Autodesk Inventor part; units mm, degrees
ref_plane "YZ Plane" through (0, 0, 0) normal (1, 0, 0) x (0, 1, 0)
ref_plane "XZ Plane" through (0, 0, 0) normal (0, 1, 0) x (-1, 0, 0)
ref_plane "XY Plane" through (0, 0, 0) normal (0, 0, 1) x (1, 0, 0)
sketch "Sketch1" plane through (0, 0, 0) normal (0, 1, 0) x (-1, 0, 0)
  line L0 (0, 0) -> (83.3, 0)
  line L1 (83.3, 0) -> (83.3, -115.6)
  line L2 (83.3, -115.6) -> (0, -115.6)
  line L3 (0, -115.6) -> (0, 0)
  dimension "d0" = 115.6
  dimension "d1" = 83.3
extrude "Lid Body" add sketch "Sketch1" along normal blind 6
fillet "4mm Fillet" radius 4 4 edges at (0, 3, -115.6) (-83.3, 3, -115.6) (-83.3, 3, 0) (0, 3, 0)
sketch "Sketch2" plane through (0, 6, 0) normal (0, 1, 0) x (1, 0, 0)
  circle A0 centre (-80.3, 3) radius 1.5
  line L0 (-83.3, 115.6) -> (-83.3, 0)
  line L1 (-83.3, 0) -> (0, 0)
  line L2 (-83.3, 57.8) -> (0, 57.8)
  line L3 (0, 0) -> (0, 115.6)
  line L4 (-41.65, 0) -> (-41.65, 124)
  circle A1 centre (-80.3, 112.6) radius 1.5
  circle A2 centre (-3, 3) radius 1.5
  circle A3 centre (-3, 112.6) radius 1.5
  dimension "d5" = 3
  dimension "d6" = 3
  dimension "d7" = 3
extrude "3mm Mounting Holes" cut sketch "Sketch2" against normal through all contours A0 | A1 | A2 | A3
sketch "Sketch3" plane through (0, 6, 0) normal (0, 1, 0) x (1, 0, 0)
  line L0 (-83.3, 0) -> (0, 0)
  line L1 (0, 0) -> (0, 115.6)
  line L2 (0, 115.6) -> (-83.3, 115.6)
  line L3 (-83.3, 115.6) -> (-83.3, 0)
  line L4 (-78.3, 5) -> (-5, 5)
  line L5 (-5, 5) -> (-5, 110.6)
  line L6 (-5, 110.6) -> (-78.3, 110.6)
  line L7 (-78.3, 110.6) -> (-78.3, 5)
  line L8 (-68, 19.3) -> (-13.5, 19.3)
  line L9 (-13.5, 19.3) -> (-13.5, 96.3)
  line L10 (-13.5, 96.3) -> (-68, 96.3)
  line L11 (-68, 96.3) -> (-68, 19.3)
  dimension "d11" = 5
  dimension "d12" = 54.5
  dimension "d13" = 77
  dimension "d14" = 10.3
  dimension "d18" = 14.3
extrude "Screen Cut-Out" cut sketch "Sketch3" against normal through all contours L11 L10 L9 L8
fillet "Fillet3" radius 1 8 edges at (-82.1284, 6, -1.1716) (-41.65, 6, 0) (-1.1716, 6, -1.1716) (0, 6, -57.8) (-1.1716, 6, -114.4284) (-41.65, 6, -115.6) (-82.1284, 6, -114.4284) (-83.3, 6, -57.8)
fillet "Fillet4" radius 2 4 edges at (-40.75, 6, -19.3) (-68, 6, -57.8) (-40.75, 6, -96.3) (-13.5, 6, -57.8)
sketch "Sketch4" plane through (0, 0, 0) normal (0, -1, 0) x (1, 0, 0)
  line L0 (-68, -19.3) -> (-13.5, -19.3)
  line L1 (-13.5, -19.3) -> (-68, -19.3)
  line L2 (-68, -19.3) -> (-68, -10.3)
  line L3 (-68, -10.3) -> (-13.5, -10.3)
  line L4 (-13.5, -10.3) -> (-13.5, -19.3)
  point P0 (0, 0)
  dimension "d21" = 9
extrude "Extrusion4" cut sketch "Sketch4" against normal blind 4
properties part number "LidTest02"
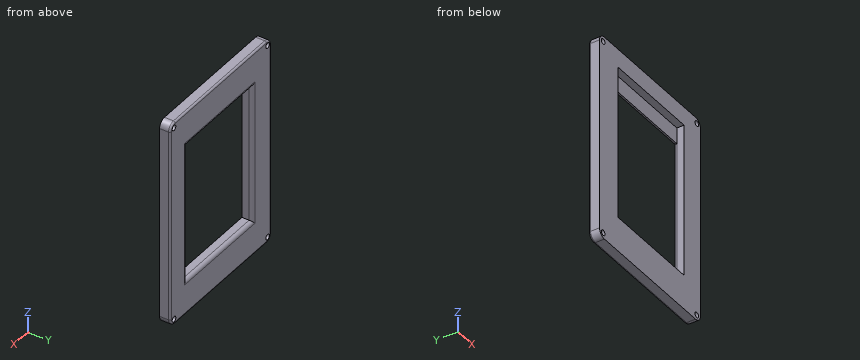
Source: CAD feature listing. Evaluate the final solid. Frame: model axes, mm. Coordinates: 2 decimals unless noted, no trailing zeros. Order: outer loops, then holes, each group sorted by start corner. A loop starts at its lowest first (then second) coordinate and runs counter-clockwise, first axis right, second up.
Item 1: Cut plane B-B (z = -38.5). Return loops of the section in (x, y), plus the area to 3 significant figures.
Output values:
outline: (-83.3, 0) - (-68, 0) - (-68, 4) arc R2 ccw to (-70, 6) - (-82.3, 6) arc R1 ccw to (-83.3, 5) - close; (-13.5, 0) - (0, 0) - (0, 5) arc R1 ccw to (-1, 6) - (-11.5, 6) arc R2 ccw to (-13.5, 4) - close
area: 171 mm2
Item 2: Cut plane A-A (x = -29.5). Return loops of the section in (y, z), plus the area to 3 significant figures.
Output values:
outline: (0, -115.6) - (5, -115.6) arc R1 ccw to (6, -114.6) - (6, -98.3) arc R2 ccw to (4, -96.3) - (0, -96.3) - close; (0, -10.3) - (4, -10.3) - (4, -19.3) arc R2 ccw to (6, -17.3) - (6, -1) arc R1 ccw to (5, 0) - (0, 0) - close
area: 193 mm2
Item 3: First-contact query: P1, Ø7, axis at x = -40.5, z = -14.5, coming from the -Y side; P2, Ø4, axis at x = -3, z = -112.6, coming from the +Y side; P3, Ø1.8, axis at x = -80.3, z = -3, coming from the +Y side. Flat tips, straight axial feed; report the tip coordinate or a pass-through.
Output values:
P1: stops at y = 4
P2: stops at y = 6
P3: passes through
Item 4: Material intervals for line 1 (Z direction, x = -46.5, y = 3.4); line 2 (X direction, y = 0.85, z = -38); line 3 (X direction, y = 2.5, z = -112.6), sorted ascending.
Output values:
line 1: z = -115.6 to -96.3, -10.3 to 0
line 2: x = -83.3 to -68, -13.5 to 0
line 3: x = -83.17 to -81.8, -78.8 to -4.5, -1.5 to -0.13
Item 5: Cut plane C-C (y = 1.9). Return loops of the section in (x, z).
Output values:
outline: (-83.3, -111.6) arc R4 ccw to (-79.3, -115.6) - (-4, -115.6) arc R4 ccw to (0, -111.6) - (0, -4) arc R4 ccw to (-4, 0) - (-79.3, 0) arc R4 ccw to (-83.3, -4) - close; hole circle Ø3 at (-80.3, -112.6); hole circle Ø3 at (-80.3, -3); hole (-68, -96.3) - (-13.5, -96.3) - (-13.5, -10.3) - (-68, -10.3) - close; hole circle Ø3 at (-3, -112.6); hole circle Ø3 at (-3, -3)
